Could you check a few things on this model? Use its own coordinates, in mm. Round coordinates to 2 decimals unless told otherwise and drop trailing zeros. Loops run counter-clockwise (first coordinate to the right, second up) from the corner with the lowest first, then second, coordinate; pieces in that order, holes last. Notation, with made-up numbers: M 62.25,41.25 L 90.25,41.25 A34 ccw 90.25,74.25 Z; hole C 29.25,14.5 d11. An arc over 180 degrees is marked long. One line per item, written item: value. Start each with the question number.
Q1. Please list where these lines run through material, in increasing order: line 1 along Y through (x, z) = (23, 4.5); line 2 along Y through (x, z) = (0, 3.5) (3 decimals); line 3 along X through (y, z) = (12.5, 5).
Q2. Imagine slicing it at C-C (z = 2.25). Please give me the cut outline in (x, y) (3 decimals), then the cut area to 3 significant figures.
Q3. I'm going to push flat-ended pins straight in: pin 1 Ø1 at (x, z) = (-9, 1.5) entering from +Y; pin 2 Ø5 at (x, y) = (23, 14) entering from -Z; pin 3 Ø2 at (x, z) = (-10, 4) entering from +Y; pin 4 Ø1 at (y, z) = (11.5, 5.5) entering from -X. Where does each tip first touch, or does it pass through?
Q4. Imagine slicing it at D-D (y = 5). Please give me the cut outline in (x, z).
Q5. Thinking about a two-plate mould opening in Y: for faces 1 (the face through (15, 19, 3)), 2 (the face through (16, 0, 7)), 3 (the face through (20.253, 0.121, 3.451)), 4 (the face through (-19, 0, 3)), which applies, released by +Y, released by -Y, zero draft, split by the parting line, or undercut?
Q6. Imagine slicing it at B-B (y = 0). Please give me the cut outline in (x, z) (3 decimals).
Q7. Imagine slicing it at A-A (x = 23). Please give me the cut outline in (y, z), then the cut area to 4 significant figures.
from build123d import *

# Parameters (mm, degrees)
SKETCH1_R           = 14.275
SKETCH1_R_2         = 2.75
BOSS_EXTRUDE1_DEPTH = 7


with BuildPart() as part:
    # Sketch1 → Boss-Extrude1 (new body)
    with BuildSketch(Plane.XY):
        with BuildLine():
            Line((0, -19), (30, -19))
            Line((30, -19), (30, 19))
            Line((30, 19), (0, 19))
            ThreePointArc((0, 19), (-19, 0), (0, -19))
        make_face()
        Circle(SKETCH1_R, mode=Mode.SUBTRACT)
        with Locations((23, 14)):
            Circle(SKETCH1_R_2, mode=Mode.SUBTRACT)
        with Locations((23, 0)):
            Circle(SKETCH1_R_2, mode=Mode.SUBTRACT)
        with Locations((23, -14)):
            Circle(SKETCH1_R_2, mode=Mode.SUBTRACT)
    extrude(amount=BOSS_EXTRUDE1_DEPTH)


solid = part.part
Report:
1. line 1: y = -19 to -16.75, -11.25 to -2.75, 2.75 to 11.25, 16.75 to 19
1. line 2: y = -19 to -14.275, 14.275 to 19
1. line 3: x = -14.31 to -6.89, 6.89 to 20.7, 25.3 to 30
2. outline: M 0,-19 L 30,-19 L 30,19 L 0,19 A19 ccw Z; hole C 0,0 d28.55; hole C 23,-14 d5.5; hole C 23,0 d5.5; hole C 23,14 d5.5
2. area: 996 mm²
3. pin 1: stops at y = 16.99
3. pin 2: passes through
3. pin 3: stops at y = 16.73
3. pin 4: stops at x = -15.49
4. outline: M -18.33,0 L -13.37,0 L -13.37,7 L -18.33,7 Z; M 13.37,0 L 30,0 L 30,7 L 13.37,7 Z
5. face 1: released by +Y
5. face 2: zero draft
5. face 3: undercut
5. face 4: split by the parting line
6. outline: M -19,0 L -14.275,0 L -14.275,7 L -19,7 Z; M 14.275,0 L 20.25,0 L 20.25,7 L 14.275,7 Z; M 25.75,0 L 30,0 L 30,7 L 25.75,7 Z
7. outline: M -19,0 L -16.75,0 L -16.75,7 L -19,7 Z; M -11.25,0 L -2.75,0 L -2.75,7 L -11.25,7 Z; M 2.75,0 L 11.25,0 L 11.25,7 L 2.75,7 Z; M 16.75,0 L 19,0 L 19,7 L 16.75,7 Z
7. area: 150.5 mm²
